```python
from build123d import *

# Parameters (mm, degrees)
SKETCH_1_R          = 1.25
SKETCH_1_R_2        = 0.5
EXTRUDE_1_DEPTH     = 2
CUT_EXTRUDE_1_REACH = 18.5
SKETCH_2_R          = 0.5
EXTRUDE_START       = 2.5
SKETCH_3_R          = 3.5
SKETCH_3_R_2        = 2.5
EXTRUDE_2_DEPTH     = 2.5


with BuildPart() as part:
    # 草圖1 → 填料-伸長1 (new body)
    with BuildSketch(Plane.XY):
        with BuildLine():
            Line((0, 3.5), (14.211482552, 1.988787352))
            ThreePointArc((14.211482552, 1.988787352), (15.997194871, -0.105889793), (14, -2))
            Line((14, -2), (0, -3.5))
            ThreePointArc((0, -3.5), (-3.5, 0), (0, 3.5))
        make_face()
        Circle(SKETCH_1_R, mode=Mode.SUBTRACT)
        with Locations((14, 0)):
            Circle(SKETCH_1_R_2, mode=Mode.SUBTRACT)
    extrude(amount=EXTRUDE_1_DEPTH)

    # 草圖2 → 除料-伸長1 (cut, up to next)
    with BuildSketch(Plane.XY.offset(2), mode=Mode.PRIVATE) as cut_extrude_1_sk1:
        with Locations((12, 0)):
            Circle(SKETCH_2_R)
    cut_extrude_1_tool1 = extrude(cut_extrude_1_sk1.sketch, amount=-CUT_EXTRUDE_1_REACH, mode=Mode.PRIVATE) & part.part
    # 草圖2 → 除料-伸長1 (cut, up to next)
    with BuildSketch(Plane.XY.offset(2), mode=Mode.PRIVATE) as cut_extrude_1_sk2:
        with Locations((10, 0)):
            Circle(SKETCH_2_R)
    cut_extrude_1_tool2 = extrude(cut_extrude_1_sk2.sketch, amount=-CUT_EXTRUDE_1_REACH, mode=Mode.PRIVATE) & part.part
    # 草圖2 → 除料-伸長1 (cut, up to next)
    with BuildSketch(Plane.XY.offset(2), mode=Mode.PRIVATE) as cut_extrude_1_sk3:
        with Locations((8, 0)):
            Circle(SKETCH_2_R)
    cut_extrude_1_tool3 = extrude(cut_extrude_1_sk3.sketch, amount=-CUT_EXTRUDE_1_REACH, mode=Mode.PRIVATE) & part.part
    # 草圖2 → 除料-伸長1 (cut, up to next)
    with BuildSketch(Plane.XY.offset(2), mode=Mode.PRIVATE) as cut_extrude_1_sk4:
        with Locations((6, 0)):
            Circle(SKETCH_2_R)
    cut_extrude_1_tool4 = extrude(cut_extrude_1_sk4.sketch, amount=-CUT_EXTRUDE_1_REACH, mode=Mode.PRIVATE) & part.part
    add(cut_extrude_1_tool1.solids().sort_by_distance((12, 0, 2))[0], mode=Mode.SUBTRACT)
    add(cut_extrude_1_tool2.solids().sort_by_distance((10, 0, 2))[0], mode=Mode.SUBTRACT)
    add(cut_extrude_1_tool3.solids().sort_by_distance((8, 0, 2))[0], mode=Mode.SUBTRACT)
    add(cut_extrude_1_tool4.solids().sort_by_distance((6, 0, 2))[0], mode=Mode.SUBTRACT)

    # 草圖3 → 填料-伸長2 (add)
    with BuildSketch(Plane(origin=(0, 0, 0), x_dir=(-1, 0, 0), z_dir=(0, 0, -1)).offset(EXTRUDE_START)):
        Circle(SKETCH_3_R)
        Circle(SKETCH_3_R_2, mode=Mode.SUBTRACT)
    extrude(amount=-EXTRUDE_2_DEPTH)


solid = part.part
```
Can you work these out from the model? Positions are in its coordinate system, mm. A direction names the side the tool comes from. Coordinates: 2 decimals unless noted, no trailing zeros. Loops run counter-clockwise (first coordinate to the right, second up) from the corner with the lowest first, then second, coordinate; pieces in that order, holes last.
1) I need wall thicknesses on probe 1 along Z at (x, y) = (3.5, 0.75); probe 2 along Y at (x, z) = (14, 1.3); probe 3 along Y at (x, z) = (9.75, 1.5). Which ranges of each line are inside material? Lowest first, please.
2) Imagine slicing it at C-C on z = -2.15. List the corners of the cut face in (x, y) for me, plus the area to 3 significant figures.
3) Imagine slicing it at D-D on y = 1.5. List the corners of the cut face in (x, z) for me.
4) Which directions (+Z, -Z, +X, -X, +Y, -Y) give clear straight access to the entire face, cutting with the end or side of a thin tool? Please do faces 1 (the cylindrical face through (-3.086, -1.651, 0.219)), 2 (the flat face through (-2, -2, -2.5)).
5) For pin 1 (1 mm diameter, centred on y = 1.5, z = -1.5, fed in from +X); pin 2 (1 mm diameter, centred on y = -1, z = 0.5, fed in from -X); pin 3 (1.5 mm diameter, centred on x = -0.5, y = 1, fed in from -Z); pin 4 (1.5 mm diameter, centred on x = 0, y = 0, fed in from -Z), each with a flat end and sliding along its axis, tell me the tip position at first contact or that it passes through.
6) Imagine slicing it at A-A on z = 0.4. List the corners of the cut face in (x, y) for me, plus the area to 3 significant figures.
Completed:
1. probe 1: z = 0 to 2
1. probe 2: y = -2 to -0.5, 0.5 to 2.01
1. probe 3: y = -2.46 to -0.43, 0.43 to 2.46
2. outline: circle Ø7 at (0, 0); hole circle Ø5 at (0, 0)
2. area: 18.8 mm2
3. outline: (-3.16, -2.5) - (-2, -2.5) - (-2, 0) - (2, 0) - (2, -2.5) - (3.16, -2.5) - (3.16, 0) - (15.32, 0) - (15.32, 2) - (-3.16, 2) - close
4. face 1: -Z
4. face 2: -Z, +X, -X, +Y, -Y
5. pin 1: stops at x = 3.35
5. pin 2: stops at x = -3.46
5. pin 3: stops at z = 0
5. pin 4: passes through
6. outline: (0, -3.5) - (14, -2) arc R2 ccw to (14.21, 1.99) - (0, 3.5) arc R3.5 ccw to start; hole circle Ø2.5 at (0, 0); hole circle Ø1 at (6, 0); hole circle Ø1 at (8, 0); hole circle Ø1 at (10, 0); hole circle Ø1 at (12, 0); hole circle Ø1 at (14, 0)
6. area: 93.8 mm2
